Autodesk Inventor part; units mm, degrees
ref_plane "Work Plane1" through (6, 0, 0) normal (1, 0, 0) x (0, 1, 0)
ref_plane "Work Plane2" through (-6, 0, 0) normal (1, 0, 0) x (0, 1, 0)
ref_plane "Work Plane3" through (10, 0, 0) normal (1, 0, 0) x (0, 1, 0)
sketch "Sketch1" plane through (0, 0, 0) normal (0, 1, 0) x (-1, 0, 0)
  circle A0 centre (0, 0) radius 20
  dimension "d0" = 40
extrude "Extrusion1" add sketch "Sketch1" along normal blind 30
sketch "Sketch2" plane through (0, 30, 0) normal (0, 1, 0) x (1, 0, 0)
  circle A0 centre (0, 0) radius 10
  dimension "d3" = 20
extrude "Extrusion2" add sketch "Sketch2" along normal blind 60
sketch "Sketch3" plane through (0, 90, 0) normal (0, 1, 0) x (1, 0, 0)
  circle A0 centre (0, 0) radius 10
  circle A1 centre (0, 0) radius 10
  circle A2 centre (0, 0) radius 6
  dimension "d6" = 20
  dimension "d7" = 12
extrude "Extrusion3" cut sketch "Sketch3" against normal blind 16
sketch "Sketch4" plane through (0, 0, 0) normal (0, -1, 0) x (1, 0, 0)
  circle A0 centre (0, 0) radius 2
  line L0 (1.5, 1.3229) -> (1.5, -1.3229)
  dimension "d10" = 4
  dimension "d11" = 3.5
extrude "Extrusion4" cut sketch "Sketch4" against normal blind 10 contours L0 A0 picked at (-0.0779, 0.6608)
fillet "Fillet1" radius 7 1 edges at (-10, 30, 0)
fillet "Fillet2" radius 7 1 edges at (20, 30, 0)
fillet "Fillet3" radius 4 1 edges at (-6, 90, 0)
ref_plane "Work Plane1" through (6, 0, 0) normal (1, 0, 0) x (0, 1, 0)
ref_plane "Work Plane2" through (-6, 0, 0) normal (1, 0, 0) x (0, 1, 0)
ref_plane "Work Plane3" through (10, 0, 0) normal (1, 0, 0) x (0, 1, 0)
sketch "Sketch7" plane through (10, 0, 0) normal (1, 0, 0) x (0, 1, 0)
  line L0 (57, 6.8) -> (37.3, 6.8)
  line L1 (37.3, 6.8) -> (37.3, -6.8)
  line L2 (37.3, -6.8) -> (57, -6.8)
  line L3 (57, -6.8) -> (57, 6.8)
  line L4 (-9.9161, 0) -> (11.1387, 0)
  line L5 (74, 10) -> (74, -10)
  line L6 (37.3, -6.8) -> (32.3, -6.8)
  line L7 (37.3, 4) -> (31.3, 4)
  line L8 (31.3, 4) -> (31.3, -4)
  line L9 (31.3, -4) -> (37.3, -4)
  line L10 (37.3, -4) -> (37.3, 4)
  point P0 (0, 0)
  dimension "d26" = 6.8
  dimension "d27" = 13.6
  dimension "d28" = 19.7
  dimension "d29" = 17
  dimension "d30" = 0
  dimension "d31" = 5
  dimension "d32" = 6
  dimension "d33" = 8
  dimension "d38" = 4
  dimension "d39" = 0
extrude "Extrusion6" cut sketch "Sketch7" along normal blind 2 and the other way blind 4
ref_plane "Work Plane4" through (12, 31.3, 4) normal (0.7071, 0.7071, 0) x (0, 0, -1)
sketch "Sketch8" plane through (12, 31.3, 4) normal (0.7071, 0.7071, 0) x (0, 0, -1)
  line L0 (8, 4.2426) -> (8, 0)
  line L1 (8, 4.3868) -> (0, 4.3868)
  line L2 (0, 4.3868) -> (0, -12.1132)
  line L3 (0, -12.1132) -> (8, -12.1132)
  line L4 (8, -12.1132) -> (8, 4.3868)
  ellipse E0 centre (4, 26.6579) end of major axis (14, 26.6579) minor radius 7.0711 (-2.8, 21.4733) -> (10.8, 21.4733) ccw
  point P0 (4, -13.6472)
  point P1 (8, 4.2426)
  dimension "d41" = 8
  dimension "d42" = 16.5
  dimension "d52" = 22.2711
extrude "Extrusion7" cut sketch "Sketch8" along normal blind 3 and the other way blind 4.2
ref_plane "Work Plane5" through (0, 0, 6) normal (0, 0, 1) x (1, 0, 0)
sketch "Sketch9" plane through (0, 0, 6) normal (0, 0, 1) x (1, 0, 0)
  circle A0 centre (0, 79) radius 1.5
  line L0 (-10, 74) -> (10, 74)
  point P0 (0, 0)
  dimension "d48" = 3
  dimension "d49" = 5
extrude "Extrusion8" cut sketch "Sketch9" against normal blind 3
mirror "Mirror2" about plane through (0, 0, 0) normal (0, 0, 1) of "Extrusion8"
sketch "Sketch10" plane through (0, 0, 0) normal (0, -1, 0) x (1, 0, 0)
  circle A0 centre (0, 0) radius 9.5
  dimension "d53" = 19
extrude "Extrusion9" cut sketch "Sketch10" against normal blind 12
sketch "Sketch11" plane through (0, 0, 0) normal (0, -1, 0) x (1, 0, 0)
  circle A0 centre (0, 0) radius 9.5
  circle A1 centre (0, 0) radius 11.5
  dimension "d56" = 23
extrude "Extrusion10" cut sketch "Sketch11" against normal blind 6.5
ref_plane "Work Plane6" through (-20, 0, 0) normal (1, 0, 0) x (0, 1, 0)
sketch "Sketch12" plane through (-20, 0, 0) normal (1, 0, 0) x (0, 1, 0)
  line L0 (0, -20) -> (0, 20)
  line L1 (0, -11.1927) -> (6.5, -11.1927)
  line L2 (6.5, -11.1927) -> (6.5, 10.8073)
  line L3 (6.5, 10.8073) -> (0, 10.8073)
  line L4 (0, 10.8073) -> (0, -11.1927)
  circle A0 centre (3.25, 0) radius 1.95
  circle A1 centre (8.75, 0) radius 1.95
  point P0 (0, 0)
  dimension "d60" = 22
  dimension "d61" = 3.9
  dimension "d62" = 6.5
  dimension "d63" = 3.25
  dimension "d64" = 0
  dimension "d65" = 3.9
  dimension "d66" = 5.5
extrude "Extrusion11" cut sketch "Sketch12" along normal blind 18 contours A0 | A1
sketch "Sketch13" plane through (-20, 0, 0) normal (1, 0, 0) x (0, 1, 0)
  line L0 (0, -4) -> (13, -4)
  line L1 (13, -4) -> (13, 4)
  line L2 (13, 4) -> (0, 4)
  line L3 (0, 4) -> (0, -4)
  point P0 (0, 0)
  dimension "d70" = 8
  dimension "d71" = 4
  dimension "d72" = 13
extrude "Extrusion12" cut sketch "Sketch13" along normal blind 2
sketch "Sketch14" plane through (0, 12, 0) normal (0, -1, 0) x (1, 0, 0)
  circle A0 centre (0, 0) radius 6.2
  line L0 (0, 0) -> (7.6867, 0)
  line L1 (0, 0) -> (-3.9527, 6.8463)
  line L2 (0, 0) -> (-3.8209, -6.618)
  circle A1 centre (-3.1, 5.3694) radius 1.45
  circle A2 centre (-3.1, -5.3694) radius 1.45
  circle A3 centre (6.2, 0) radius 1.45
  dimension "d75" = 12.4
  dimension "d76" = 120
  dimension "d77" = 120
  dimension "d79" = 2.9
  dimension "d80" = 2.9
  dimension "d81" = 2.9
extrude "Extrusion13" cut sketch "Sketch14" against normal blind 12 contours L0 A3 A0 | L0 A3 A0 | A0 A3 L0 | A0 A3 L0 | A1 L1 A0 | A0 L1 A1 | A2 A0 | A0 L2 A2 | L1 A1 A0 | A0 A1 L1 | A0 A2 L2
sketch "Sketch15" plane through (0, 0, 0) normal (1, 0, 0) x (0, 1, 0)
  line L0 (95, -20.5708) -> (0, -20.5708)
  line L1 (0, -20.5708) -> (0, 21.1406)
  line L2 (0, 21.1406) -> (95, 21.1406)
  line L3 (95, 21.1406) -> (95, -20.5708)
  line L4 (20, -20.5708) -> (20, 21.1406)
  point P0 (0, 0)
  dimension "d84" = 20
  dimension "d85" = 41.7114
  dimension "d86" = 95
extrude "Extrusion14" cut sketch "Sketch15" along normal mid plane 40 contours L0 L4 L2 L3
sketch "Sketch16" plane through (0, 20, 0) normal (0, 1, 0) x (1, 0, 0)
  line L0 (18.2415, 4.1496) -> (17.0061, 4.1496)
  line L1 (17.0061, 4.1496) -> (17.0061, -4.2806)
  line L2 (17.0061, -4.2806) -> (18.2415, -4.2806)
  line L3 (18.2415, -4.2806) -> (18.2415, 4.1496)
  point P0 (0, 0)
extrude "Extrusion15" add sketch "Sketch16" against normal blind 3
sketch "Sketch17" plane through (0, 20, 0) normal (0, 1, 0) x (1, 0, 0)
  circle A0 centre (0, 0) radius 15
  circle A1 centre (-3.1, -5.3694) radius 1.45
  circle A2 centre (-3.1, -5.3694) radius 4
  circle A3 centre (-3.1, 5.3694) radius 1.45
  circle A4 centre (-3.1, 5.3694) radius 4
  circle A5 centre (6.2, 0) radius 1.45
  circle A6 centre (6.2, 0) radius 4
  dimension "d91" = 30
  dimension "d92" = 8
  dimension "d93" = 8
  dimension "d94" = 8
extrude "Extrusion16" cut sketch "Sketch17" against normal blind 4 contours A2 | A4 | A6
sketch "Sketch18" plane through (0, 20, 0) normal (0, 1, 0) x (1, 0, 0)
  circle A0 centre (0, 0) radius 15
  line L0 (0, 0) -> (18.2122, 0)
  line L1 (0, 0) -> (-8.7364, -15.1318)
  line L2 (0, 0) -> (-8.9499, 15.5016)
  circle A1 centre (15, 0) radius 1.5
  circle A2 centre (-7.5, -12.9904) radius 1.5
  circle A3 centre (-7.5, 12.9904) radius 1.5
  dimension "d97" = 30
  dimension "d98" = 120
  dimension "d99" = 120
  dimension "d100" = 3
  dimension "d101" = 3
  dimension "d102" = 3
extrude "Extrusion17" cut sketch "Sketch18" against normal blind 40 contours L0 A1 A0 | L0 A1 A0 | A0 A1 L0 | A0 A1 L0 | A3 L2 A0 | A0 L2 A3 | A2 L1 A0 | A0 L1 A2 | L2 A3 A0 | A0 A3 L2 | L1 A2 A0 | A0 A2 L1
sketch "Sketch19" plane through (0, 0, 0) normal (0, -1, 0) x (1, 0, 0)
  circle A0 centre (-7.5, -12.9904) radius 1.5
  circle A1 centre (-7.5, -12.9904) radius 3.5
  circle A2 centre (15, 0) radius 1.5
  circle A3 centre (15, 0) radius 3.5
  circle A4 centre (-7.5, 12.9904) radius 1.5
  circle A5 centre (-7.5, 12.9904) radius 3.5
  point P0 (0, 0)
  dimension "d105" = 7
  dimension "d106" = 7
  dimension "d107" = 7
extrude "Extrusion18" cut sketch "Sketch19" against normal blind 5
properties part number "EF1"
Build history of the part. All positions in model axes, mm. A direction names the side the tool comes from. Give positions to 0.01 mm unless a question says otherwise; leave off trailing zeros. Loops run counter-clockwise (first coordinate to the right, second up) from the corner with the lowest first, then second, coordinate; pieces in that order, holes last. Notation, with made-up numbers: (-11, 7.5) -> (12, 7.5) arc R14 cw to (12, 13.5) -> close; hole circle Ø10 at (76, 6). An arc over 180 degrees is marked (long way). One line per question, with ' | ' between items.
Q1. Cut at B-B, the plane x = 15. Write the cut outline in (y, z), plus the area to 3 significant figures.
Filled sheet:
outline: (0, -13.23) -> (20, -13.23) -> (20, -1.5) -> (5, -1.5) -> (5, -3.5) -> (0, -3.5) -> close; (0, 3.5) -> (5, 3.5) -> (5, 1.5) -> (20, 1.5) -> (20, 13.23) -> (0, 13.23) -> close | area: 449 mm²
Q2. Drill centre lines: line 1 along Y through (x, z) = (-14, 0); line 2 along Z through (x, y) = (-7.5, 1.4); line 3 along Z through (x, y) = (0.5, 2). Where is each one in solid material? Low to high. Write a range as [from, to].
Filled sheet:
line 1: y = [0, 1.3], [5.2, 6.8], [10.7, 20] | line 2: z = [-18.54, -16.49], [-9.49, -8.72], [8.72, 9.49], [16.49, 18.54] | line 3: z = [-19.99, -11.49], [11.49, 19.99]
Q3. Drop flat-ended pins along their axis: pin 1 (0.5 mm diameter, centred on x = -18.5, y = 6.5, fed in from +Z); pin 2 (2 mm diameter, centred on x = -6.5, z = -12.5, fed in from -Y); pin 3 (3 mm diameter, centred on x = -12, z = -8, fed in from -Y); pin 4 (3.5 mm diameter, centred on y = 8.75, z = 0, fed in from -X). Give the stop position or say it passes through.
Filled sheet:
pin 1: stops at z = 8.18 | pin 2: stops at y = 5 | pin 3: stops at y = 0 | pin 4: stops at x = 9.34
Q4. Cut at A-A, the plane z = 6. Write the cut outline in (x, y), plus the area to 3 significant figures.
Filled sheet:
outline: (-19.08, 0) -> (-9.81, 0) -> (-9.81, 6.5) -> (-7.37, 6.5) -> (-7.37, 12) -> (-4.41, 12) -> (-4.41, 16) -> (-7.05, 16) -> (-7.05, 20) -> (-19.08, 20) -> close; (-1.79, 12) -> (7.37, 12) -> (7.37, 6.5) -> (9.81, 6.5) -> (9.81, 0) -> (19.08, 0) -> (19.08, 20) -> (0.85, 20) -> (0.85, 16) -> (-1.79, 16) -> close | area: 513 mm²
Q5. Tool access for faces 4 (the cylindrical face through (8.776, 9.212, -3.639)), 5 (the flat face through (-1, 16, 5)), 6 (the flat face through (-18, 6, 0)), 7 (the cylindrical face through (-14.71, 5.11, -0.59)): list every direction of +Z, -Z, +X, -X, +Y, -Y with a clear straight run to the whole face (end or side of a thin tool).
Filled sheet:
face 4: -Y | face 5: +Y | face 6: -X, -Y | face 7: -X
Q6. Cut at D-D, the plane x = -3.1. Write the cut outline in (y, z), plus the area to 3 significant figures.
Filled sheet:
outline: (0, -19.76) -> (20, -19.76) -> (20, -9.37) -> (16, -9.37) -> (16, -6.82) -> (12, -6.82) -> (12, -8.98) -> (6.5, -8.98) -> (6.5, -11.07) -> (0, -11.07) -> close; (0, 11.07) -> (6.5, 11.07) -> (6.5, 8.98) -> (12, 8.98) -> (12, 6.82) -> (16, 6.82) -> (16, 9.37) -> (20, 9.37) -> (20, 19.76) -> (0, 19.76) -> close; (12, -3.92) -> (16, -3.92) -> (16, -1.37) -> (20, -1.37) -> (20, 1.37) -> (16, 1.37) -> (16, 3.92) -> (12, 3.92) -> close | area: 460 mm²
Q7. Pull direction Z, two halves, no side cores. Call faces 1 (the cylindrical face through (4.336, 9.86, 19.524)), 2 (the flat face through (0, 20, 0)), 3 (the flat face through (-19, 13, 0)): pulls with the +Z half, pulls with the -Z half, needs draft (parallel to the pull), parting line crosses it, or undercut.
Filled sheet:
face 1: parting line crosses it | face 2: needs draft | face 3: undercut
